The model under review builds one solid part; all positions refer to its coordinate system, in mm. A direction names the side the tool comes from. Round coordinates to 2 decimals unless told otherwise and drop trailing zeros. Order: outer loops, then holes, each group sorted by start corner. A loop starts at its lowest first (then second) coordinate and runs counter-clockwise, first axis right, second up. Notation, with made-up numbers: M 10.5,83 L 34.5,83 A14 ccw 34.5,97 Z; hole C 67,7.25 d11. An arc over 180 degrees is marked long. Use a Markdown table: item, result. Add a question column.
1. For faces 1 (the flat face through (35, 1.5, 1)), 2 (the flat face through (-15, -1, -1)), list the 3-axis set-ups (+Z, -Z, +X, -X, +Y, -Y) from which the entire face can be reached by the end or side of a thin tool; tool diameter is ignored.
2. To check wall thickness, follow probe 1 along Z at (x, y) = (-10.5, -1.8); probe 2 along Y at (x, z) = (-26, -5); probe 3 along Z at (x, y) = (-30.5, 0.8). State the ranges of each line that lie inside material, in increasing order.
3. Consider section C-C on x = 16.5. State the section outline as (y, z) points.
4. Consider section B-B on y = -0.65. State the section outline as (x, z) points, then the cut area to 3 significant figures.
5. Insertion check: P1, Ø1, axis at x = -10, z = -9, coming from the -Y side; P2, Ø1.5, axis at y = -0.5, z = -15.5, coming from the -X side. Each pin has a flat end and moves straight along its axis. Give the tip position at first contact, or say it passes through.
6. Consider section A-A on x = -14. State the section outline as (y, z) points.
from build123d import *

# Parameters (mm, degrees)
BOSS_EXTRUDE1_DEPTH = 1.5
SKETCH2_W           = 1
SKETCH2_H           = 36
CUT_EXTRUDE1_DEPTH  = 0.5
SKETCH3_W           = 30
SKETCH3_H           = 2
BOSS_EXTRUDE2_DEPTH = 2
CHAMFER1_SIZE       = 0.5


with BuildPart() as part:
    # Sketch1 → Boss-Extrude1 (new body)
    with BuildSketch(Plane(origin=(0, 0, 0), x_dir=(1, 0, 0), z_dir=(0, 1, 0))):
        Polygon((-38.5, 8.06761956), (-26.5, 20.06761956), (26.5, 20.06761956), (38.5, 8.06761956), (38.5, -15.93238044), (-38.5, -15.93238044), align=None)
    extrude(amount=BOSS_EXTRUDE1_DEPTH)

    # Sketch2 → Cut-Extrude1 (cut)
    with BuildSketch(Plane(origin=(0, 1.5, 0), x_dir=(1, 0, 0), z_dir=(0, 1, 0))):
        with Locations((-36.5, 2.06761956)):
            Rectangle(SKETCH2_W, SKETCH2_H)
        with Locations((-33.458333333, 2.06761956)):
            Rectangle(SKETCH2_W, SKETCH2_H)
        with Locations((-30.416666667, 2.06761956)):
            Rectangle(SKETCH2_W, SKETCH2_H)
        with Locations((-27.375, 2.06761956)):
            Rectangle(SKETCH2_W, SKETCH2_H)
        with Locations((-24.333333333, 2.06761956)):
            Rectangle(SKETCH2_W, SKETCH2_H)
        with Locations((-21.291666667, 2.06761956)):
            Rectangle(SKETCH2_W, SKETCH2_H)
        with Locations((-18.25, 2.06761956)):
            Rectangle(SKETCH2_W, SKETCH2_H)
        with Locations((-15.208333333, 2.06761956)):
            Rectangle(SKETCH2_W, SKETCH2_H)
        with Locations((-12.166666667, 2.06761956)):
            Rectangle(SKETCH2_W, SKETCH2_H)
        with Locations((-9.125, 2.06761956)):
            Rectangle(SKETCH2_W, SKETCH2_H)
        with Locations((-6.083333333, 2.06761956)):
            Rectangle(SKETCH2_W, SKETCH2_H)
        with Locations((-3.041666667, 2.06761956)):
            Rectangle(SKETCH2_W, SKETCH2_H)
        with Locations((0, 2.06761956)):
            Rectangle(SKETCH2_W, SKETCH2_H)
        with Locations((3.041666667, 2.06761956)):
            Rectangle(SKETCH2_W, SKETCH2_H)
        with Locations((6.083333333, 2.06761956)):
            Rectangle(SKETCH2_W, SKETCH2_H)
        with Locations((9.125, 2.06761956)):
            Rectangle(SKETCH2_W, SKETCH2_H)
        with Locations((12.166666667, 2.06761956)):
            Rectangle(SKETCH2_W, SKETCH2_H)
        with Locations((15.208333333, 2.06761956)):
            Rectangle(SKETCH2_W, SKETCH2_H)
        with Locations((18.25, 2.06761956)):
            Rectangle(SKETCH2_W, SKETCH2_H)
        with Locations((21.291666667, 2.06761956)):
            Rectangle(SKETCH2_W, SKETCH2_H)
        with Locations((24.333333333, 2.06761956)):
            Rectangle(SKETCH2_W, SKETCH2_H)
        with Locations((27.375, 2.06761956)):
            Rectangle(SKETCH2_W, SKETCH2_H)
        with Locations((30.416666667, 2.06761956)):
            Rectangle(SKETCH2_W, SKETCH2_H)
        with Locations((33.458333333, 2.06761956)):
            Rectangle(SKETCH2_W, SKETCH2_H)
        with Locations((36.5, 2.06761956)):
            Rectangle(SKETCH2_W, SKETCH2_H)
    extrude(amount=-CUT_EXTRUDE1_DEPTH, mode=Mode.SUBTRACT)

    # Sketch3 → Boss-Extrude2 (add)
    with BuildSketch(Plane.XZ):
        with Locations((0, -1.06761956)):
            Rectangle(SKETCH3_W, SKETCH3_H)
    extrude(amount=BOSS_EXTRUDE2_DEPTH)

    # Chamfer1
    chamfer1_edges = [part.edges().sort_by_distance(p)[0] for p in [
        (36, 1, 2.68238044),
        (32.958333333, 1, 1.161547107),
        (37, 1, 3.18238044),
        (33.958333333, 1, 1.661547107),
        (30.916666667, 1, 0.140713774),
        (27.875, 1, -1.38011956),
        (24.833333333, 1, -2.06761956),
        (21.791666667, 1, -2.06761956),
        (18.75, 1, -2.06761956),
        (15.708333333, 1, -2.06761956),
        (29.916666667, 1, -0.359286226),
        (26.875, 1, -1.88011956),
        (23.833333333, 1, -2.06761956),
        (20.791666667, 1, -2.06761956),
        (17.75, 1, -2.06761956),
        (14.708333333, 1, -2.06761956),
        (11.666666667, 1, -2.06761956),
        (8.625, 1, -2.06761956),
        (5.583333333, 1, -2.06761956),
        (2.541666667, 1, -2.06761956),
        (12.666666667, 1, -2.06761956),
        (9.625, 1, -2.06761956),
        (6.583333333, 1, -2.06761956),
        (3.541666667, 1, -2.06761956),
        (0.5, 1, -2.06761956),
        (-2.541666667, 1, -2.06761956),
        (-5.583333333, 1, -2.06761956),
        (-8.625, 1, -2.06761956),
        (-11.666666667, 1, -2.06761956),
        (-14.708333333, 1, -2.06761956),
        (-17.75, 1, -2.06761956),
        (-20.791666667, 1, -2.06761956),
        (-0.5, 1, -2.06761956),
        (-3.541666667, 1, -2.06761956),
        (-6.583333333, 1, -2.06761956),
        (-9.625, 1, -2.06761956),
        (-12.666666667, 1, -2.06761956),
        (-15.708333333, 1, -2.06761956),
        (-18.75, 1, -2.06761956),
        (-21.791666667, 1, -2.06761956),
        (-24.833333333, 1, -2.06761956),
        (-27.875, 1, -1.38011956),
        (-23.833333333, 1, -2.06761956),
        (-26.875, 1, -1.88011956),
        (-29.916666667, 1, -0.359286226),
        (-30.916666667, 1, 0.140713774),
        (-33.958333333, 1, 1.661547107),
        (-32.958333333, 1, 1.161547107),
        (-36, 1, 2.68238044),
        (-37, 1, 3.18238044),
    ]]
    chamfer(chamfer1_edges, length=CHAMFER1_SIZE - 0.0001)  # a hair under: the kernel refuses the full size


solid = part.part
Answer block:
| question | item | result |
|---|---|---|
| 1 | face 1 | +Z, -Z, +X, -X, +Y |
| 1 | face 2 | +Z, -Z, -X, -Y |
| 2 | probe 1 | -2.07 to -0.07 |
| 2 | probe 2 | 0 to 1.5 |
| 2 | probe 3 | -16.07 to 15.93 |
| 3 | outline | M 0,-20.07 L 1.5,-20.07 L 1.5,15.93 L 0,15.93 Z |
| 4 | outline | M -15,-2.07 L 15,-2.07 L 15,-0.07 L -15,-0.07 Z |
| 4 | area | 60.0 mm^2 |
| 5 | P1 | y = 0 |
| 5 | P2 | x = -31.63 |
| 6 | outline | M -2,-2.07 L 0,-2.07 L 0,-20.07 L 1.5,-20.07 L 1.5,15.93 L 0,15.93 L 0,-0.07 L -2,-0.07 Z |
